Check sheet for the modelled part. Datum: model origin and axes. Units: mm. A direction names the side the tool comes from. Round coordinates to 2 decimals unless told otherwise and drop trailing zeros. Loops run counter-clockwise (first coordinate to the right, second up) from the corner with the lowest first, then second, coordinate; pieces in that order, holes last. Notation, with made-up numbers: (35.5, -12.75) -> (54.5, -12.75) arc R10 cw to (54.5, 4.25) -> close; hole circle Ø7 at (36.25, 39). An arc over 180 degrees is marked (long way). Return JSON: item names as keys, results as strings.
from build123d import *

# Parameters (mm, degrees)
SKETCH1_W           = 90
SKETCH1_H           = 380
SKETCH1_W_2         = 2.2
SKETCH1_H_2         = 8.1
BOSS_EXTRUDE1_DEPTH = 21
CUT_EXTRUDE1_DEPTH  = 99.352414984
SKETCH2_W           = 3
SKETCH2_H           = 360
BOSS_EXTRUDE2_DEPTH = 40


with BuildPart() as part:
    # Sketch1 → Boss-Extrude1 (new body)
    with BuildSketch(Plane(origin=(0, 0, 0), x_dir=(1, 0, 0), z_dir=(0, 1, 0))):
        Rectangle(SKETCH1_W, SKETCH1_H)
        with Locations((46.1, 185.95)):
            Rectangle(SKETCH1_W_2, SKETCH1_H_2)
        Polygon((49.24, 178), (47.2, 178), (47.2, 193.9), (49.24, 193.9), (53.352414984, 189.998), (53.352414984, 181.902), align=None)
    extrude(amount=BOSS_EXTRUDE1_DEPTH)

    # Sketch3 → Cut-Extrude1 (cut, through all)
    with BuildSketch(Plane.ZY.offset(45)):
        Polygon((190, 0), (-160, 21), (190, 21), align=None)
    extrude(amount=-CUT_EXTRUDE1_DEPTH, mode=Mode.SUBTRACT)

    # Sketch2 → Boss-Extrude2 (add)
    with BuildSketch(Plane.XZ):
        with Locations((-46.5, 10)):
            Rectangle(SKETCH2_W, SKETCH2_H)
    boss_extrude2 = extrude(amount=-BOSS_EXTRUDE2_DEPTH)

    # Mirror1: Boss-Extrude2 across plane
    add(boss_extrude2.mirror(Plane(origin=(0, 0, 0), x_dir=(0, 0, 1), z_dir=(1, 0, 0))))


solid = part.part
Q1. Section check D-D (x = -24). Record the boundary of the cut face in (y, z), then the cut area to 4 significant figures.
Results list:
{"outline": "(0, -190) -> (21, -190) -> (21, -160) -> (0, 190) -> close", "area": "4,305 mm^2"}
Q2. Section check C-C (y = 15). Record the boundary of the cut face in (x, z).
Results list:
{"outline": "(-48, -170) -> (-45, -170) -> (-45, -190) -> (47.2, -190) -> (47.2, -193.9) -> (49.24, -193.9) -> (53.35, -190) -> (53.35, -181.9) -> (49.24, -178) -> (47.2, -178) -> (47.2, -181.9) -> (45, -181.9) -> (45, -170) -> (48, -170) -> (48, 190) -> (45, 190) -> (45, -60) -> (-45, -60) -> (-45, 190) -> (-48, 190) -> close"}
Q3. Draft check along X on faces 4 (the flat face through (45, 10, -176)), 5 (the flat face through (2, 10, -190)), 6 (the flat face through (-45, 10, -180)). Enter one of: released by +X, released by -X, zero draft, split by the parting line, or undercut.
Results list:
{"face 4": "undercut", "face 5": "zero draft", "face 6": "released by -X"}
Q4. Go/stop test with flat-tipped pins: pin 1 (2 mm diameter, centred on y = 6.5, z = -191.5, fed in from -X); pin 2 (6 mm diameter, centred on y = 14.5, z = -176, fed in from -X); pin 3 (1.5 mm diameter, centred on y = 6.5, z = 19, fed in from +X). Record where each tip stops, or that it passes through.
Results list:
{"pin 1": "x = 47.2", "pin 2": "x = -45", "pin 3": "x = 48"}
Q5. Material ranges on line 1 (X direction, y = 28, z = -80); line 2 (X direction, y = 7, z = -22); line 3 (Y direction, x = 28.5, z = -159.5), recorded low to high.
Results list:
{"line 1": "-48 to -45, 45 to 48", "line 2": "-48 to 48", "line 3": "0 to 20.97"}
Q6. Section check A-A (y = 33.5). Record the boundary of the cut face in (x, z), then the cut area to 3 significant figures.
Results list:
{"outline": "(-48, -170) -> (-45, -170) -> (-45, 190) -> (-48, 190) -> close; (45, -170) -> (48, -170) -> (48, 190) -> (45, 190) -> close", "area": "2,160 mm^2"}
Q7. Tool access check on faces 1 (the flat face through (48, 20, 7)), 2 (the flat face through (-0.63, 10.353, 17.45)), 3 (the flat face through (-48, 20, 7)). Record the directions out of +Z, -Z, +X, -X, +Y, -Y that give a thin tool (end or side, any length) a straight path to the whole face; none if there is none.
Results list:
{"face 1": "+Z, +X, +Y, -Y", "face 2": "+Z, +Y", "face 3": "+Z, -Z, -X, +Y, -Y"}
Q8. Section check B-B (z = 104). Record the boundary of the cut face in (x, y).
Results list:
{"outline": "(-48, 0) -> (48, 0) -> (48, 40) -> (45, 40) -> (45, 5.16) -> (-45, 5.16) -> (-45, 40) -> (-48, 40) -> close"}
